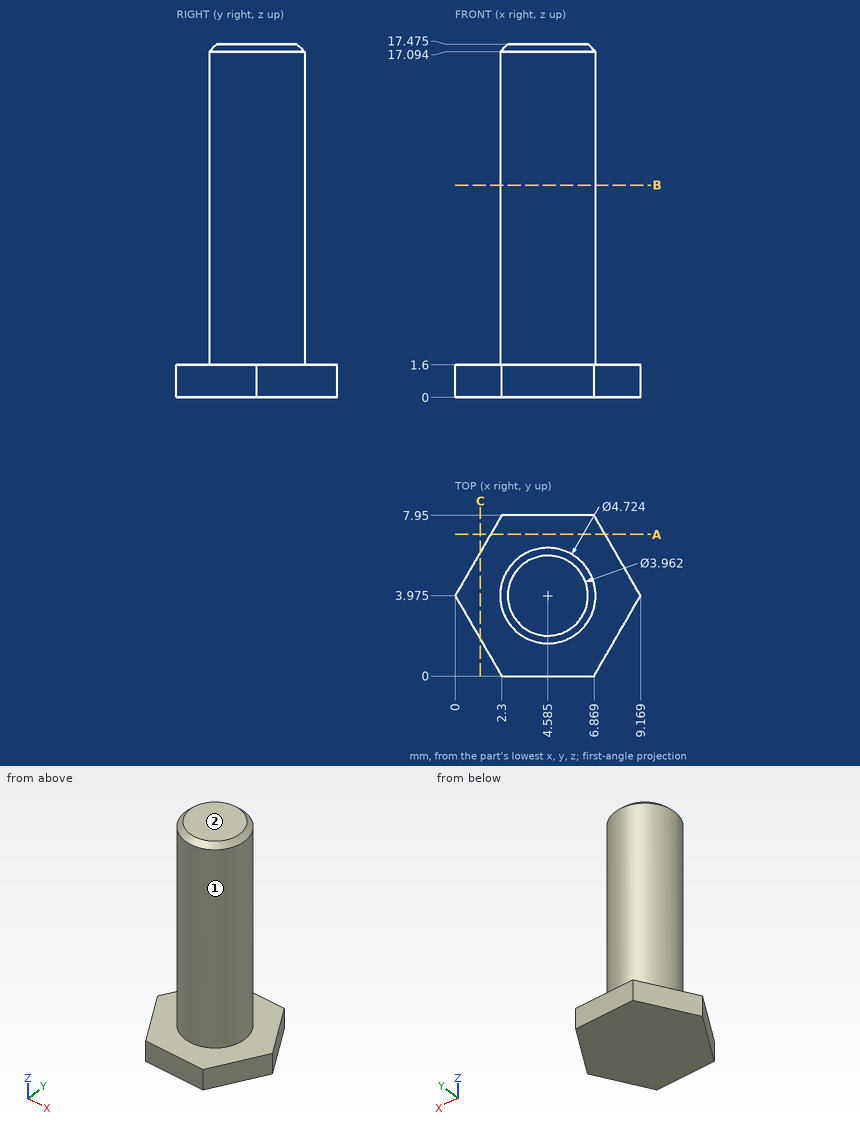
The figure shows three views and two pictorial views of one solid part (mm, origin at its lowest corner). Answer the questions. A direction names the side the tool comes from. Coordinates: 2 decimals unless noted, no trailing zeros. Write each loop counter-clockwise with the first axis right and the second up, starting at its lowest first coordinate (ties: lowest second). Pieces come first, ordered by that corner, then holes. Notation, with made-up numbers: (-34, 35) -> (-1, 35) arc R20 ccw to (-1, 50) -> close; hole circle Ø8 at (61.5, 72). An arc over 180 degrees is marked (long way). Answer as a JSON object with one key per item and string values.
Q1. Consider line 1 (Z direction, x = 6.75, y = 5.5); line 2 (Y direction, x = 4.5, z = 13.5) (1 decimal); line 3 (Y direction, x = 6.75, z = 4) (1 decimal). Determine where each line is inside the solid, lowest interval first. Write a range as [from, to].
The answers:
{"line 1": "z = [0, 1.6]", "line 2": "y = [1.6, 6.3]", "line 3": "y = [3, 4.9]"}
Q2. A tool of negligible diameter and unlimited length cuts with its end or side. For the marked faces 1 and 2, from which of +Z, -Z, +X, -X, +Y, -Y can it reach the whole face along a straight path? Write none if from no direction.
The answers:
{"face 1": "+Z", "face 2": "+Z, +X, -X, +Y, -Y"}
Q3. The part is cut by section C-C on x = 1.25. Give the vertices of the cut face in (y, z) (1 decimal).
The answers:
{"outline": "(1.8, 0) -> (6.1, 0) -> (6.1, 1.6) -> (1.8, 1.6) -> close"}
Q4. Flat-ended cylindrical pins translate along their axes: pin 1 Ø2 at (x, z) = (4, 9.5) entering from +Y; pin 2 Ø1 at (y, z) = (1.5, 9) entering from +X; pin 3 Ø2 at (y, z) = (2.5, 14) entering from -X. Find the tip coordinate at first contact, or state that the pin passes through.
The answers:
{"pin 1": "stops at y = 6.34", "pin 2": "stops at x = 5.88", "pin 3": "stops at x = 2.27"}
Q5. The part is cut by section B-B on z = 10.5. Give the vertices of the cut face in (x, y) (1 decimal), then the cut area to 3 significant figures.
The answers:
{"outline": "circle Ø4.7 at (4.6, 4)", "area": "17.5 mm2"}
Q6. The part is cut by section A-A on y = 7. Give the vertices of the cut face in (x, z).
The answers:
{"outline": "(1.75, 0) -> (7.42, 0) -> (7.42, 1.6) -> (1.75, 1.6) -> close"}
